Could you check a few things on this model? Use its own coordinates, in mm. Give positions to 0.01 mm unless a question says otherwise; leave off trailing zeros. Write each loop counter-clockwise with the first axis right and the second up, starting at its lowest first coordinate (ties: lowest second). Pieces come first, ordered by that corner, then holes. Notation, with made-up numbers: M -24.5,-4 L -10.5,-4 A15 ccw -10.5,17 Z; hole C -9,87.5 d3. An arc over 180 degrees is marked long. Use one line per item in the form item = value.
from build123d import *

# Parameters (mm, degrees)
SKIZZE1_W                       = 145
SKIZZE1_H                       = 156
AUFSATZ_LINEAR_AUSTRAGEN1_DEPTH = 3
DURCHGANGSLOCH_F_R_M41_D        = 4.5
DURCHGANGSLOCH_F_R_M41_DEPTH    = 3
DURCHGANGSLOCH_F_R_M41_TIP      = 1.351936393
SKIZZE5_W                       = 50
SKIZZE5_H                       = 23
SCHNITT_LINEAR_AUSTRAGEN1_DEPTH = 107.532858781


with BuildPart() as part:
    # Skizze1 → Aufsatz-Linear austragen1 (new body)
    with BuildSketch(Plane.XY):
        Rectangle(SKIZZE1_W, SKIZZE1_H)
    extrude(amount=AUFSATZ_LINEAR_AUSTRAGEN1_DEPTH)

    # Durchgangsloch für M41
    with Locations(Plane.XY.offset(3)):
        with Locations((25, 66), (-47.5, -66), (47.5, -66)):
            Hole(DURCHGANGSLOCH_F_R_M41_D / 2, depth=DURCHGANGSLOCH_F_R_M41_DEPTH)
            with Locations((0, 0, -(DURCHGANGSLOCH_F_R_M41_DEPTH + DURCHGANGSLOCH_F_R_M41_TIP / 2))):  # 118° drill point
                Cone(0, DURCHGANGSLOCH_F_R_M41_D / 2, DURCHGANGSLOCH_F_R_M41_TIP, mode=Mode.SUBTRACT)

    # Skizze5 → Schnitt-Linear austragen1 (cut, through all)
    with BuildSketch(Plane(origin=(0, 0, 0), x_dir=(-1, 0, 0), z_dir=(0, 0, -1))):
        with Locations((47.5, 66.5)):
            Rectangle(SKIZZE5_W, SKIZZE5_H)
    extrude(amount=-SCHNITT_LINEAR_AUSTRAGEN1_DEPTH, mode=Mode.SUBTRACT)


solid = part.part
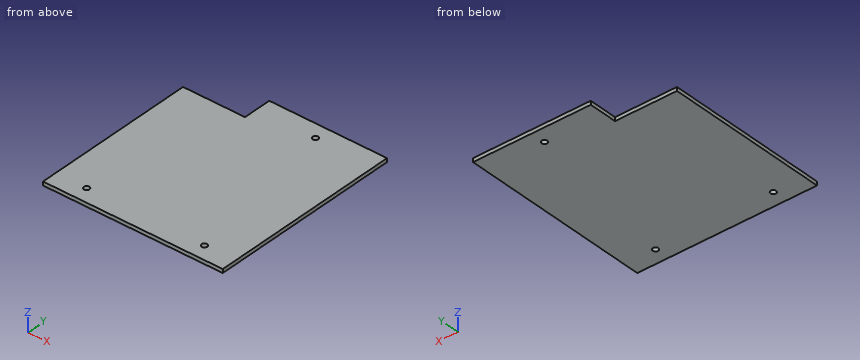
1) I want a section at A-A, the plane x = -47.5. Please give me the cut outline in (y, z), plus the area to 4 significant figures.
Checked values:
outline = M -78,0 L -68.25,0 L -68.25,3 L -78,3 Z; M -63.75,0 L 55,0 L 55,3 L -63.75,3 Z
area = 385.5 mm2
2) If I drill on L1, parallel to X at y = 66, z = 1.65; L2, parallel to X at y = -66, z = 1.75; L3, parallel to Y at x = 47.5, z = 1.2, over which ranges is the centre line in solid material (lowest first)?
Checked values:
L1 = -22.5 to 22.75, 27.25 to 72.5
L2 = -72.5 to -49.75, -45.25 to 45.25, 49.75 to 72.5
L3 = -78 to -68.25, -63.75 to 78
3) I want a section at B-B, the plane y = -66. Please give me the cut outline in (x, z), plus the area to 3 significant figures.
Checked values:
outline = M -72.5,0 L -49.75,0 L -49.75,3 L -72.5,3 Z; M -45.25,0 L 45.25,0 L 45.25,3 L -45.25,3 Z; M 49.75,0 L 72.5,0 L 72.5,3 L 49.75,3 Z
area = 408 mm2
4) I want a section at C-C, the plane y = 66. Please give me the cut outline in (x, z), plus the area to 4 significant figures.
Checked values:
outline = M -22.5,0 L 22.75,0 L 22.75,3 L -22.5,3 Z; M 27.25,0 L 72.5,0 L 72.5,3 L 27.25,3 Z
area = 271.5 mm2
5) For pin 1 Ø0.9 at (y, z) = (67.5, 2) entering from -X; pin 2 Ø1 at (x, z) = (-43.5, 1.5) entering from +Y, each with a flat end and sliding along its axis, tell me the tip position at first contact or that it passes through.
Checked values:
pin_1 = -22.5
pin_2 = 55
